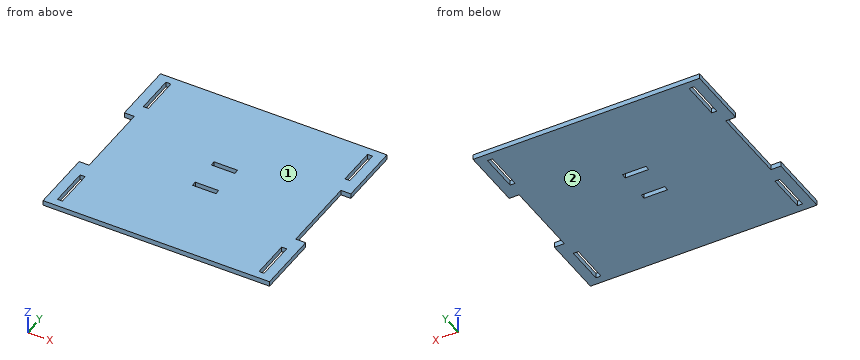
from build123d import *

# Parameters (mm, degrees)
SKETCH1_W           = 3.175
SKETCH1_H           = 25
SKETCH1_W_2         = 15
SKETCH1_H_2         = 3.175
BOSS_EXTRUDE1_DEPTH = 3.175


with BuildPart() as part:
    # Sketch1 → Boss-Extrude1 (new body)
    with BuildSketch(Plane.XY):
        Polygon((0, 90), (6.35, 90), (6.35, 40), (0, 40), (0, 0), (144.35, 0), (144.35, 40), (138, 40), (138, 90), (144.35, 90), (144.35, 130), (0, 130), align=None)
        with Locations((7.9375, 112.5)):
            Rectangle(SKETCH1_W, SKETCH1_H, mode=Mode.SUBTRACT)
        with Locations((136.4125, 112.5)):
            Rectangle(SKETCH1_W, SKETCH1_H, mode=Mode.SUBTRACT)
        with Locations((7.9375, 17.5)):
            Rectangle(SKETCH1_W, SKETCH1_H, mode=Mode.SUBTRACT)
        with Locations((136.4125, 17.5)):
            Rectangle(SKETCH1_W, SKETCH1_H, mode=Mode.SUBTRACT)
        with Locations((72.175, 54.5875)):
            Rectangle(SKETCH1_W_2, SKETCH1_H_2, mode=Mode.SUBTRACT)
        with Locations((72.175, 75.4125)):
            Rectangle(SKETCH1_W_2, SKETCH1_H_2, mode=Mode.SUBTRACT)
    extrude(amount=BOSS_EXTRUDE1_DEPTH)


solid = part.part
Geometry: final body of the model. Coordinates: model frame, mm. Face numbers are marked on the shaded views. Give positions to 0.01 mm unless a question says otherwise; leave off trailing zeros. Write each loop counter-clockwise with the first axis right and the second up, starting at its lowest first coordinate (ties: lowest second). Pieces come first, ordered by that corner, then holes. Notation, with made-up numbers: (32, -2) - (44, -2) arc R21 cw to (44, 10) - close; hole circle Ø6 at (27.25, -23.75). An arc over 180 degrees is marked (long way). Return JSON: item names as keys, results as strings. Group by question number.
1) Section D-D on y = 79.5. Return the cut outline in (x, z) (3 decimals), plus the area to 3 significant figures.
2) Mould query, pull axis Z, two halves, no side actions, for the marked faces 1 and 2. Classes: released by +Z, released by -Z, zero draft, split by the parting line, or undercut.
3) Section A-A on x = 72. Return the cut outline in (y, z) (3 decimals).
4) Section C-C on z = 2.25. State how many separate pieces and enclosed holes the cut face has, plus the area to 3 significant figures.
5) First-contact query: P1, Ø1, axis at y = 54, z = 1, coming from the +X side; P2, Ø1, axis at y = 63, z = 2.5, coming from the -X side. Flat tips, straight axial feed; report the tip coordinate or a pass-through.
6) Section B-B on y = 19.5. Return the cut outline in (x, z) (3 decimals), plus the area to 3 significant figures.
7) Line query: line 1 (X direction, y = 16, z = 2.3) (3 decimals); line 2 (Y direction, x = 135, z = 2.2); line 3 (X direction, y = 50.5, z = 2.3). Output: solid intervals per line, ascending.
Filled in:
{
 "1": {"outline": "(6.35, 0) - (138, 0) - (138, 3.175) - (6.35, 3.175) - close", "area": "418 mm^2"},
 "2": {"face 1": "released by +Z", "face 2": "released by -Z"},
 "3": {"outline": "(0, 0) - (53, 0) - (53, 3.175) - (0, 3.175) - close; (56.175, 0) - (73.825, 0) - (73.825, 3.175) - (56.175, 3.175) - close; (77, 0) - (130, 0) - (130, 3.175) - (77, 3.175) - close"},
 "4": {"separate pieces": "1", "enclosed holes": "6", "area": "17,700 mm^2"},
 "5": {"P1": "stops at x = 138", "P2": "stops at x = 6.35"},
 "6": {"outline": "(0, 0) - (6.35, 0) - (6.35, 3.175) - (0, 3.175) - close; (9.525, 0) - (134.825, 0) - (134.825, 3.175) - (9.525, 3.175) - close; (138, 0) - (144.35, 0) - (144.35, 3.175) - (138, 3.175) - close", "area": "438 mm^2"},
 "7": {"line 1": "x = 0 to 6.35, 9.525 to 134.825, 138 to 144.35", "line 2": "y = 0 to 5, 30 to 100, 125 to 130", "line 3": "x = 6.35 to 138"}
}
